Work out the finished part from the listing and answer in its coordinate system (mm). A direction names the side the tool comes from. Round coordinates to 2 decimals unless told otherwise and drop trailing zeros. Loops run counter-clockwise (first coordinate to the right, second up) from the corner with the lowest first, then second, coordinate; pieces in that order, holes last.
Autodesk Inventor part; units mm, degrees
ref_plane "YZ Plane" through (0, 0, 0) normal (1, 0, 0) x (0, 1, 0)
ref_plane "XZ Plane" through (0, 0, 0) normal (0, 1, 0) x (-1, 0, 0)
ref_plane "XY Plane" through (0, 0, 0) normal (0, 0, 1) x (1, 0, 0)
sketch "Sketch1" plane through (0, 0, 0) normal (0, 0, 1) x (1, 0, 0)
  line L0 (-42.5241, -5.0241) -> (236.8759, -5.0241)
  line L1 (97.1759, -5.0241) -> (97.1759, 52.1259)
  line L2 (97.1759, 52.1259) -> (-4.4241, 52.1259)
  line L3 (-4.4241, 52.1259) -> (198.7759, 52.1259)
  line L4 (198.7759, 52.1259) -> (236.8759, -5.0241)
  line L5 (-4.4241, 52.1259) -> (-42.5241, -5.0241)
  point P0 (0, 0)
  dimension "d0" = 279.4
  dimension "d1" = 57.15
  dimension "d2" = 101.6
  dimension "d3" = 203.2
extrude "Extrusion1" add sketch "Sketch1" along normal blind 38.1
sketch "Sketch2" plane through (0, 0, 0) normal (0, 0, -1) x (-1, 0, 0)
  line L0 (-236.8759, -5.0241) -> (-198.7759, 52.1259)
  line L1 (42.5241, -5.0241) -> (-236.8759, -5.0241)
  line L2 (4.4241, 52.1259) -> (42.5241, -5.0241)
  line L3 (-198.7759, 52.1259) -> (4.4241, 52.1259)
  line L4 (23.4741, 23.5509) -> (-217.8259, 23.5509)
  line L5 (-97.1759, -5.0241) -> (-97.1759, 52.1259)
  circle A0 centre (-97.1759, 23.5509) radius 9.525
  point P0 (0, 0)
  dimension "d6" = 19.05
extrude "Extrusion2" add sketch "Sketch2" along normal blind 12.7 contours A0 L5 L4 | L4 L5 A0 | L5 L4 A0 | L5 A0 L4
sketch "Sketch3" plane through (97.1759, 23.5509, -12.7) normal (0, 0, -1) x (-1, 0, 0)
  circle A0 centre (0, 0) radius 9.525
  line L0 (0, 0) -> (-44.45, 0)
  line L1 (-44.45, 0) -> (-44.45, -34.925)
  line L2 (-44.45, -34.925) -> (44.45, -34.925)
  line L3 (44.45, -34.925) -> (44.45, 34.925)
  line L4 (44.45, 34.925) -> (-44.45, 34.925)
  line L5 (-44.45, 0) -> (-44.45, 34.925)
  point P0 (97.1759, -23.5509)
  dimension "d9" = 44.45
  dimension "d10" = 34.925
  dimension "d11" = 88.9
  dimension "d12" = 69.85
extrude "Extrusion3" add sketch "Sketch3" along normal blind 25.4 contours A0 | L5 L4 L3 L2 L1
sketch "Sketch4" plane through (-42.5241, -5.0241, 0) normal (0, -1, 0) x (1, 0, 0)
  line L0 (0, 0) -> (279.4, 0)
  line L1 (279.4, 0) -> (279.4, 38.1)
  line L2 (139.7, 0) -> (139.7, 19.05)
  line L3 (139.7, 19.05) -> (152.4, 19.05)
  line L4 (152.4, 19.05) -> (139.7, 19.05)
  line L5 (139.7, 19.05) -> (127, 19.05)
  circle A0 centre (127, 19.05) radius 9.525
  circle A1 centre (152.4, 19.05) radius 9.525
  line L6 (139.7, 19.05) -> (76.2, 19.05)
  circle A2 centre (76.2, 19.05) radius 9.525
  point P0 (42.5241, 0)
  dimension "d15" = 12.7
  dimension "d16" = 12.7
  dimension "d17" = 12.7
  dimension "d18" = 19.05
  dimension "d19" = 19.05
  dimension "d20" = 63.5
extrude "Extrusion4" cut sketch "Sketch4" against normal blind 2.54
sketch "Sketch5" plane through (0, 0, 0) normal (0, 0, -1) x (-1, 0, 0)
  circle A0 centre (-97.1759, 23.5509) radius 9.525
  line L0 (-198.7759, 52.1259) -> (4.4241, 52.1259)
  line L1 (-97.1759, 23.5509) -> (0.8241, 23.5509)
  line L2 (-97.1759, 23.5509) -> (-195.1759, 23.5509)
  circle A1 centre (-195.1759, 23.5509) radius 2.3813
  circle A2 centre (0.8241, 23.5509) radius 2.3813
  point P0 (0, 0)
  dimension "d23" = 98
  dimension "d24" = 98
  dimension "d25" = 4.7625
extrude "Extrusion5" cut sketch "Sketch5" against normal blind 6.35 contours A1 | A2
properties part number "kinect basic"
1. Determine the mould class of faces 1 (the face through (195, 24, 6.35)), 2 (the face through (-23.21, 23.95, 18.78)), 3 (the face through (88, 21, -6)), 4 (the face through (34, -2.484, 19)) for opening direction X: +X half, -X half, draft (parallel to the pull), parting line (faces both ways), or undercut.
Answer key:
face 1: undercut
face 2: -X half
face 3: parting line
face 4: undercut
2. Find section B-B (z = 19.05). Write down the section's boundary in (x, y), then the cut area to 3 significant figures.
Answer key:
outline: (-42.52, -5.02) - (24.15, -5.02) - (24.15, -2.48) - (43.2, -2.48) - (43.2, -5.02) - (74.95, -5.02) - (74.95, -2.48) - (94, -2.48) - (94, -5.02) - (100.35, -5.02) - (100.35, -2.48) - (119.4, -2.48) - (119.4, -5.02) - (236.88, -5.02) - (198.78, 52.13) - (-4.42, 52.13) - close
area: 13,600 mm2
3. Which of the six approach directions +Z, -Z, +X, -X, +Y, -Y give full straight-line access (tool end or side, diameter ignored) to faces 5 (the face through (114.27, -3.77, 10.6)), 6 (the face through (-1.923, 21.438, 3.131)), 7 (the face through (141.626, 23, -25))?
Answer key:
face 5: -Y
face 6: -Z
face 7: -Z, +X, +Y, -Y
4. Consider probe 1 along Z at (x, y) = (119.5, 17.5); probe 2 along Z at (x, y) = (196, 24); probe 3 along X at (y, z) = (7.5, -23.5). Determine where each line is inside the solid, lowest interval first.
Answer key:
probe 1: z = -38.1 to -12.7, 0 to 38.1
probe 2: z = 6.35 to 38.1
probe 3: x = 52.73 to 141.63
5. Find section D-D (x = 207.5). Write down the section's boundary in (y, z), then the cut area to 3 significant figures.
Answer key:
outline: (-5.02, 0) - (39.04, 0) - (39.04, 38.1) - (-5.02, 38.1) - close
area: 1,680 mm2
6. Find section C-C (x = 169). Write down the section's boundary in (y, z).
Answer key:
outline: (-5.02, 0) - (52.13, 0) - (52.13, 38.1) - (-5.02, 38.1) - close
7. Find section A-A (x = 116). Write down the section's boundary in (y, z).
Answer key:
outline: (-11.37, -38.1) - (58.48, -38.1) - (58.48, -12.7) - (-11.37, -12.7) - close; (-5.02, 0) - (52.13, 0) - (52.13, 38.1) - (-5.02, 38.1) - (-5.02, 26.35) - (-2.48, 26.35) - (-2.48, 11.75) - (-5.02, 11.75) - close
8. Given pin 1 (1 mm diameter, centred on y = 2, z = -18, fed in from -X); pin 2 (3 mm diameter, centred on y = 1, z = 3.5, fed in from -X); pin 3 (21 mm diameter, centred on x = 34, z = 20, fed in from -Y), each flat-ended and moving along its own axis, determine where each tip first touches the part or whether it passes through.
Answer key:
pin 1: stops at x = 52.73
pin 2: stops at x = -39.51
pin 3: stops at y = -5.02
